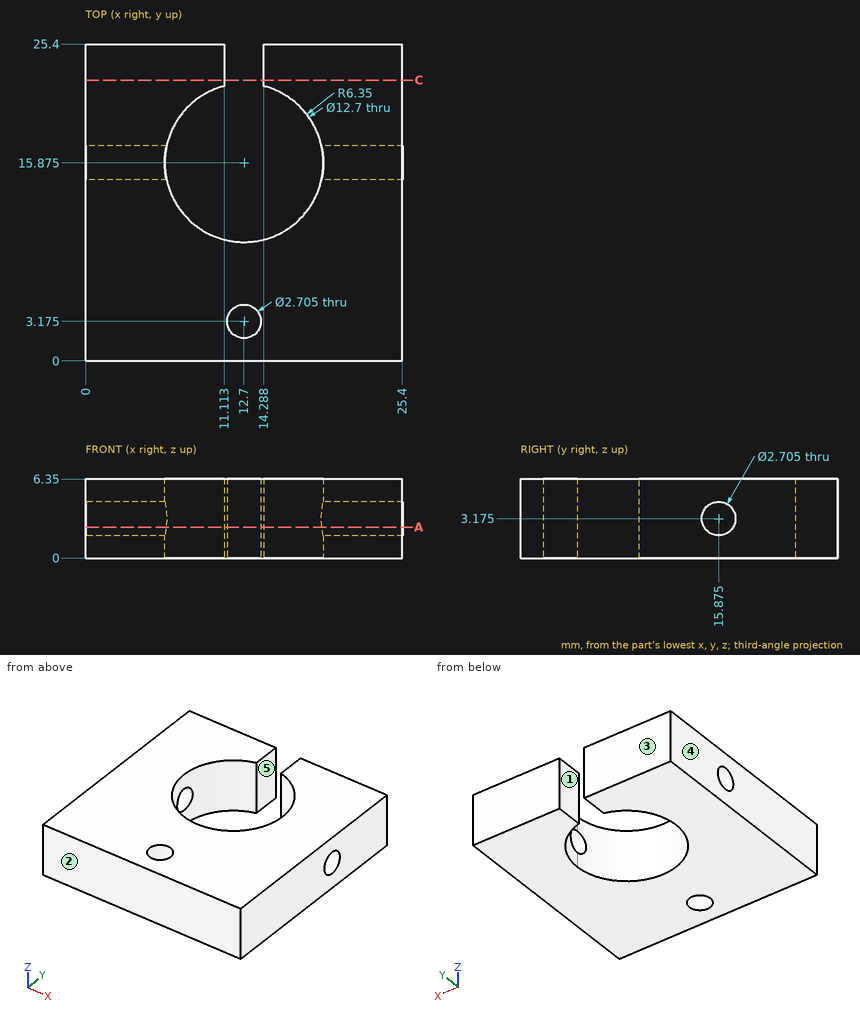
Geometry check sheet. Reference: drawing and pictorial views, mm from the part's lowest x, y, z. A direction names the side the tool comes from. Give positions to 0.01 mm unless a question says otherwise; leave off trailing zeros. Order: outer loops, then holes, each group sorted by start corner. A loop starts at its lowest first (then second) coordinate and runs counter-clockwise, first axis right, second up.
1. Access from +Z, -Z, +X, -X, +Y, -Y to the whole of each face (thin tool, end or side, straight path). Record for the marked faces 1 and 2.
2. Section check C-C, the plane y = 22.5. Enter the section's corners in (x, z).
3. Release check for a two-part mould opening along X. For the marked faces 3, 4 and 5 record: pulls with the +X half, pulls with the -X half, needs draft (parallel to the pull), parting line crosses it, or undercut.
4. Thickness scan on L1, parallel to X at y = 23.75, z = 6; L2, parallel to X at y = 2.75, z = 1.75 (1 decimal); L3, parallel to Y at x = 11.75, z = 2 (1 decimal). Record the ranges inside material, lowest first.
5. Section check A-A, the plane z = 2.5. Give the number of separate pieces and of enclosed holes in the cut face.
Values follow:
1. face 1: +Z, -Z, +Y
1. face 2: +Z, -Z, +X, -X, -Y
2. outline: (0, 0) - (11.11, 0) - (11.11, 6.35) - (0, 6.35) - close; (14.29, 0) - (25.4, 0) - (25.4, 6.35) - (14.29, 6.35) - close
3. face 3: needs draft
3. face 4: pulls with the -X half
3. face 5: undercut
4. L1: x = 0 to 11.11, 14.29 to 25.4
4. L2: x = 0 to 11.4, 14 to 25.4
4. L3: y = 0 to 2.2, 4.1 to 9.6
5. separate pieces: 3
5. enclosed holes: 1
